```python
from build123d import *

# Parameters (mm, degrees)
SKETCH1_W              = 100
SKETCH1_H              = 140
BASE_FLANGE1_DEPTH     = 1
SKETCHED_START         = -140
SKETCHED_BEND1_DEPTH   = 140
SKETCHED_BEND1_2_DEPTH = 140
CUT_EXTRUDE1_REACH     = 158.698
CUT_EXTRUDE2_REACH     = 181.598
SKETCH17_W             = 11.2
SKETCH17_H             = 22.8


# Read off the part's stored shape, not the designer's step: Sketched Bend1
# Sheet-metal steps are written as plain solids
with BuildPart() as part:
    # Sketch1 → Base-Flange1 (new body)
    with BuildSketch(Plane(origin=(0, 0, 0), x_dir=(1, 0, 0), z_dir=(0, 1, 0))):
        with Locations((50, 70)):
            Rectangle(SKETCH1_W, SKETCH1_H)
    extrude(amount=-BASE_FLANGE1_DEPTH)

    # Sketched Bend1 outline → Sketched Bend1 (cut)
    with BuildSketch(Plane.XY.offset(SKETCHED_START)):
        with BuildLine():
            ThreePointArc((51.7366, -1), (50.804773836, -0.728828115), (50.16395891, 0))
            Line((50.16395891, 0), (0, 0))
            Line((0, 0), (0, -1))
            Line((0, -1), (51.7366, -1))
        make_face()
    extrude(amount=SKETCHED_BEND1_DEPTH, mode=Mode.SUBTRACT)

    # Sketched Bend1 2 outline → Sketched Bend1 2 (add)
    with BuildSketch(Plane.XY.offset(SKETCHED_START)):
        with BuildLine():
            Line((51, 50.530753262), (50, 50.530753262))
            Line((50, 50.530753262), (50, 0.7366))
            ThreePointArc((50, 0.7366), (50.041485243, 0.359286442), (50.16395891, 0))
            Line((50.16395891, 0), (51.7366, 0))
            ThreePointArc((51.7366, 0), (51.215745145, 0.215745145), (51, 0.7366))
            Line((51, 0.7366), (51, 50.530753262))
        make_face()
    extrude(amount=SKETCHED_BEND1_2_DEPTH)

    # Sketch14 → Cut-Extrude1 (cut, up to next)
    with BuildSketch(Plane(origin=(51, 0, 0), x_dir=(0, 0, -1), z_dir=(1, 0, 0)), mode=Mode.PRIVATE) as cut_extrude1_sk1:
        with BuildLine():
            Line((13, 38.030753262), (13, 13.030753262))
            ThreePointArc((13, 13.030753262), (9.5, 9.530753262), (6, 13.030753262))
            Line((6, 13.030753262), (6, 38.030753262))
            ThreePointArc((6, 38.030753262), (9.5, 41.530753262), (13, 38.030753262))
        make_face()
    cut_extrude1_tool1 = extrude(cut_extrude1_sk1.sketch, amount=-CUT_EXTRUDE1_REACH, mode=Mode.PRIVATE) & part.part
    # Sketch14 → Cut-Extrude1 (cut, up to next)
    with BuildSketch(Plane(origin=(51, 0, 0), x_dir=(0, 0, -1), z_dir=(1, 0, 0)), mode=Mode.PRIVATE) as cut_extrude1_sk2:
        with BuildLine():
            Line((127, 38.030753262), (127, 13.030753262))
            ThreePointArc((127, 13.030753262), (130.5, 9.530753262), (134, 13.030753262))
            Line((134, 13.030753262), (134, 38.030753262))
            ThreePointArc((134, 38.030753262), (130.5, 41.530753262), (127, 38.030753262))
        make_face()
    cut_extrude1_tool2 = extrude(cut_extrude1_sk2.sketch, amount=-CUT_EXTRUDE1_REACH, mode=Mode.PRIVATE) & part.part
    add(cut_extrude1_tool1.solids().sort_by_distance((51, 25.530753, -9.5))[0], mode=Mode.SUBTRACT)
    add(cut_extrude1_tool2.solids().sort_by_distance((51, 25.530753, -130.5))[0], mode=Mode.SUBTRACT)

    # Sketch17 → Cut-Extrude2 (cut, up to next)
    with BuildSketch(Plane.XZ.offset(1), mode=Mode.PRIVATE) as cut_extrude2_sk1:
        with Locations((78, -44.4)):
            Rectangle(SKETCH17_W, SKETCH17_H)
    cut_extrude2_tool1 = extrude(cut_extrude2_sk1.sketch, amount=-CUT_EXTRUDE2_REACH, mode=Mode.PRIVATE) & part.part
    add(cut_extrude2_tool1.solids().sort_by_distance((78, -1, -44.4))[0], mode=Mode.SUBTRACT)


solid = part.part
```
Verification items for the finished model (mm, model axes). A direction names the side the tool comes from. Round coordinates to 2 decimals unless told otherwise and drop trailing zeros. Write each loop counter-clockwise with the first axis right and the second up, starting at its lowest first coordinate (ties: lowest second). Pieces come first, ordered by that corner, then holes.
1. Gauge pin test, flat ends, axial feed: P1, Ø3, axis at x = 61.5, z = -31.5, coming from the +Y side; P2, Ø0.8, axis at y = -0.5, z = -46, coming from the -X side; P3, Ø15, axis at y = 17.5, z = -50.5, coming from the +X side. Record the tip position at first contact, or that the pin passes through.
2. Scan lines: L1, parallel to Y at x = 58, z = -78; L2, parallel to X at y = 1.5, z = -13.5. Record each from-to range of solid material in increasing order.
3. Access from +Z, -Z, +X, -X, +Y, -Y to the whole of each face (thin tool, end or side, straight path). Record for faces 1 (the flat face through (76, 0, -71)), 2 (the cylindrical face through (50.51, 41.53, -9.42)), 3 (the flat face through (50.8, 24.9, -140)).
4. Section check B-B on z = -48.5. Enter the section's corners in (x, y).
5. Section check A-A on y = 22.5. Enter the section's corners in (x, z).
6. Section check C-C on x = 76. Enter the section's corners in (y, z).
7. Section check D-D on z = -85. Enter the section's corners in (x, y), plus the area to 4 significant figures.
8. Draft check along Z on faces 4 (the cylindrical face through (50.51, 9.53, -9.58)), 5 (the flat face through (51, 25, -71)), 6 (the flat face through (50.8, 24.9, 0)). Enter one of: +Z half, -Z half, draft (parallel to the pull), parting line (faces both ways), or undercut.
Answer:
1. P1: stops at y = 0
1. P2: stops at x = 50.21
1. P3: stops at x = 51
2. L1: y = -1 to 0
2. L2: x = 50 to 51
3. face 1: +Z, -Z, +X, +Y
3. face 2: +X, -X
3. face 3: -Z, +X, -X, +Y, -Y
4. outline: (50, 0.74) arc R1.74 ccw to (51.74, -1) - (72.4, -1) - (72.4, 0) - (51.74, 0) arc R0.74 cw to (51, 0.74) - (51, 50.53) - (50, 50.53) - close; (83.6, -1) - (100, -1) - (100, 0) - (83.6, 0) - close
5. outline: (50, -140) - (51, -140) - (51, -134) - (50, -134) - close; (50, -127) - (51, -127) - (51, -13) - (50, -13) - close; (50, -6) - (51, -6) - (51, 0) - (50, 0) - close
6. outline: (-1, -140) - (0, -140) - (0, -55.8) - (-1, -55.8) - close; (-1, -33) - (0, -33) - (0, 0) - (-1, 0) - close
7. outline: (50, 0.74) arc R1.74 ccw to (51.74, -1) - (100, -1) - (100, 0) - (51.74, 0) arc R0.74 cw to (51, 0.74) - (51, 50.53) - (50, 50.53) - close
7. area: 100.0 mm2
8. face 4: undercut
8. face 5: draft
8. face 6: +Z half
